The drawing under review shows one solid part. Ordinate dimensions are in mm from its lowest x, y, z. A direction names the side the tool comes from. Coordinates: 2 decimals unless noted, no trailing zeros. Loops run counter-clockwise (first coordinate to the right, second up) from the corner with the lowest first, then second, coordinate; pieces in that order, holes last. Notation, with made-up numbers: M -27,82 L 11,82 A20 cw 11,118 Z; hole C 78.5,-25.5 d3. An arc over 180 degrees is marked long. Return JSON: item names as keys, results as strings.
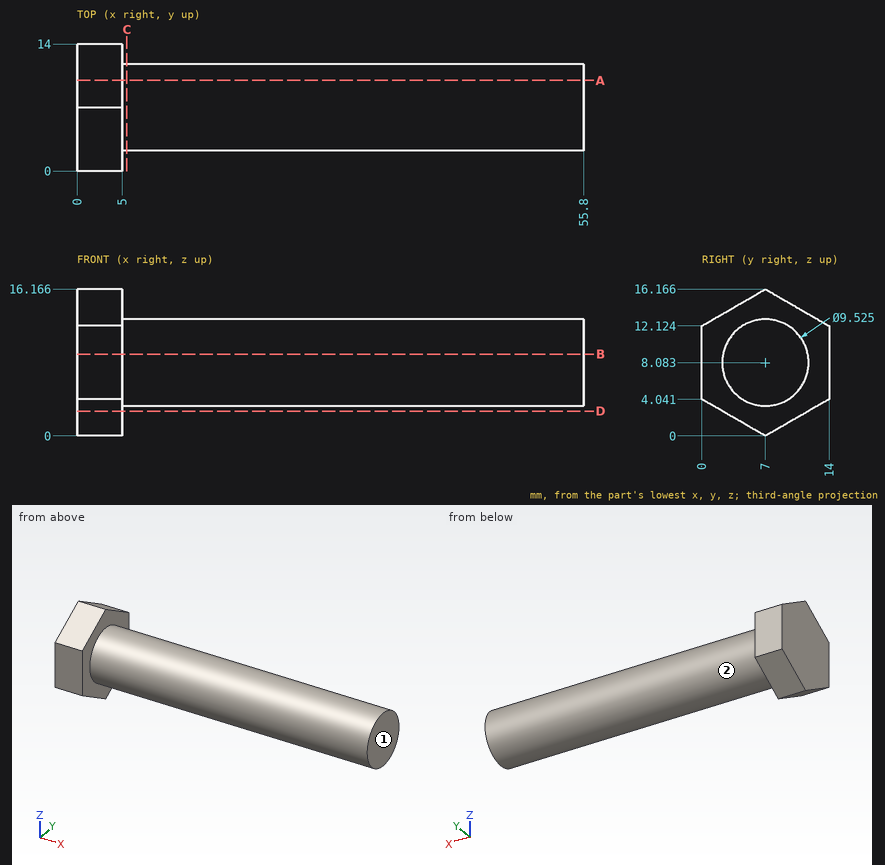
1. Add section D-D on z = 2.75. Give the boundary of the cut face in (x, y).
Check values:
{"outline": "M 0,2.24 L 5,2.24 L 5,11.76 L 0,11.76 Z"}
2. To check wall thickness, follow line 1 (X direction, y = 1.25, z = 9.5); line 2 (Z direction, x = 28, y = 2.75) (1 decimal); line 3 (Y direction, x = 28, z = 4.25) (1 decimal). State the ranges of each line that lie inside material, in increasing order.
Check values:
{"line 1": "0 to 5", "line 2": "5.9 to 10.2", "line 3": "4.2 to 9.8"}
3. Add section C-C on x = 5.5. Give the boundary of the cut face in (y, z) (1 decimal).
Check values:
{"outline": "C 7,8.1 d9.5"}
4. Machinability: for the marked faces 1 and 2, which of the approach directions +Z, -Z, +X, -X, +Y, -Y give a long, thin tool a straight path to every point of the face, cutting with its end or side? Answer none if there is none.
Check values:
{"face 1": "+Z, -Z, +X, +Y, -Y", "face 2": "+X"}
5. Add section A-A on y = 10. Give the boundary of the cut face in (x, z), plus the area to 3 significant figures.
Check values:
{"outline": "M 0,1.73 L 5,1.73 L 5,4.38 L 55.8,4.38 L 55.8,11.78 L 5,11.78 L 5,14.43 L 0,14.43 Z", "area": "439 mm²"}
6. Insertion check: pin 1 Ø2 at (x, z) = (21.5, 12.5) entering from -Y; pin 2 Ø5 at (x, z) = (22, 5) entering from -Y; pin 3 Ø5 at (x, y) = (35, 3) entering from -Z. Each pin has a flat end and moves straight along its axis. Give the tip position at first contact, or say it passes through.
Check values:
{"pin 1": "y = 3.68", "pin 2": "y = 2.27", "pin 3": "z = 3.56"}
7. Add section B-B on z = 9. Give the boundary of the cut face in (x, y), plus the area to 3 significant figures.
Check values:
{"outline": "M 0,0 L 5,0 L 5,2.33 L 55.8,2.33 L 55.8,11.67 L 5,11.67 L 5,14 L 0,14 Z", "area": "545 mm²"}
